```python
from build123d import *

# Parameters (mm, degrees)
SKETCH1_W           = 8.73
SKETCH1_H           = 8.73
BOSS_EXTRUDE1_DEPTH = 2.22
SKETCH2_R           = 25.695
BOSS_EXTRUDE2_DEPTH = 6
BOSS_EXTRUDE2_TAPER = 7
SKETCH3_R           = 23.86
CUT_EXTRUDE1_DEPTH  = 8.22
CUT_EXTRUDE1_DRAFT  = 7


with BuildPart() as part:
    # Sketch1 → Boss-Extrude1 (new body)
    with BuildSketch(Plane.XY):
        Polygon((-31.75, 0), (31.75, 0), (46.25, 25.11473671), (13.75, 81.406387956), (-13.75, 81.406387956), (-46.25, 25.11473671), align=None)
        Polygon((-34.392628869, 10.177167467), (-38.757628869, 17.737569242), (-31.197227094, 22.102569242), (-26.832227094, 14.542167467), align=None, mode=Mode.SUBTRACT)
        with Locations((0, 74.281387956)):
            Rectangle(SKETCH1_W, SKETCH1_H, mode=Mode.SUBTRACT)
        Polygon((34.392628869, 10.177167467), (38.757628869, 17.737569242), (31.197227094, 22.102569242), (26.832227094, 14.542167467), align=None, mode=Mode.SUBTRACT)
    extrude(amount=BOSS_EXTRUDE1_DEPTH)

    # Sketch2 → Boss-Extrude2 (add)
    with BuildSketch(Plane.XY.offset(2.22)):
        with Locations((0, 38)):
            Circle(SKETCH2_R)
    extrude(amount=BOSS_EXTRUDE2_DEPTH, taper=BOSS_EXTRUDE2_TAPER)


with BuildPart() as cut_extrude1_tool:
    # Sketch3 → Cut-Extrude1 (with draft: the straight prism first)
    with BuildSketch(Plane.XY.offset(8.22)):
        with Locations((0, 38)):
            Circle(SKETCH3_R)
    extrude(amount=-CUT_EXTRUDE1_DEPTH)
    # Cut-Extrude1: the draft: its side faces are tilted about the plane it starts from
    cut_extrude1_sides = [cut_extrude1_tool.faces().sort_by_distance(p)[0] for p in [
        (-23.86, 38, 4.11),
    ]]
    draft(cut_extrude1_sides, Plane.XY.offset(8.22), CUT_EXTRUDE1_DRAFT)


with BuildPart() as part_1:
    add(part.part)

    # Cut-Extrude1: cut by cut_extrude1_tool
    add(cut_extrude1_tool.part, mode=Mode.SUBTRACT)


solid = part_1.part
```
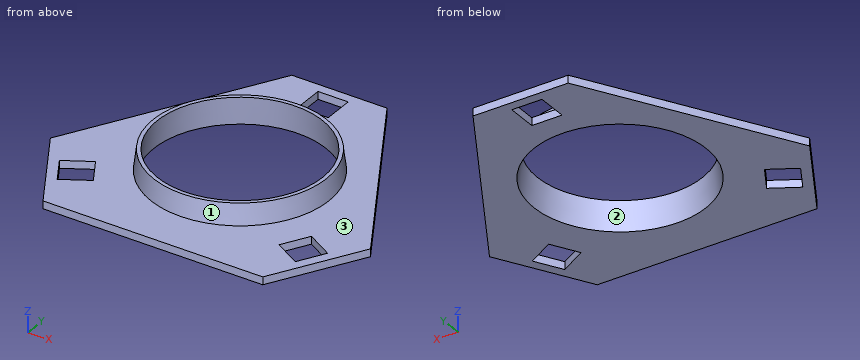
Could you check a few things on this model? Use its own coordinates, in mm. Face numbers are marked on the shaded views. Round coordinates to 2 decimals unless told otherwise and drop trailing zeros. Write each loop counter-clockwise with the first axis right and the second up, starting at its lowest first coordinate (ties: lowest second). Pieces come first, ordered by that corner, then holes.
(1) Suppose I cut it at D-D on z = 4.5. Write out the boundary of the cut face in (x, y).
Findings below:
outline: circle Ø50.83 at (0, 38); hole circle Ø48.63 at (0, 38)
(2) If I drill on probe 1 along X at (y, z) = (17.5, 1.75); probe 2 along Z at (x, y) = (17.5, 14); probe 3 along X at (y, z) = (22, 1.5), over which ranges is the centre line in solid material (lowest first)?
Findings below:
probe 1: x = -41.85 to -38.62, -28.54 to -13.7, 13.7 to 28.54, 38.62 to 41.85
probe 2: z = 0 to 2.22
probe 3: x = -44.45 to -31.37, -31.14 to -18.8, 18.8 to 31.14, 31.37 to 44.45
(3) Suppose I cut it at C-C on y = 38. Write out the boundary of the cut face in (x, z) (3 decimals), and give its area (3 significant figures).
Findings below:
outline: (-38.811, 0) - (-24.869, 0) - (-23.86, 8.22) - (-24.958, 8.22) - (-25.695, 2.22) - (-38.811, 2.22) - close; (23.86, 8.22) - (24.869, 0) - (38.811, 0) - (38.811, 2.22) - (25.695, 2.22) - (24.958, 8.22) - close
area: 75.7 mm2
(4) Suppose I cut it at A-A on x = 0. Write out the boundary of the cut face in (y, z) (3 decimals).
Findings below:
outline: (0, 0) - (13.131, 0) - (14.14, 8.22) - (13.042, 8.22) - (12.305, 2.22) - (0, 2.22) - close; (61.86, 8.22) - (62.869, 0) - (69.916, 0) - (69.916, 2.22) - (63.695, 2.22) - (62.958, 8.22) - close; (78.646, 0) - (81.406, 0) - (81.406, 2.22) - (78.646, 2.22) - close
(5) For pin 1 (1.1 mm diameter, centred on y = 75, z = 1, fed in from -X); pin 2 (8 mm diameter, centred on x = 30, y = 27, fed in from +Z); pin 3 (2.5 mm diameter, centred on y = 76, z = 1.5, fed in from +X), each with a flat end and sliding along its axis, tell me the tip position at first contact or that it passes through.
Findings below:
pin 1: stops at x = -17.77
pin 2: stops at z = 2.22
pin 3: stops at x = 17.59
(6) Thinking about a two-plate mould opening in X: for the marked faces 1, 2 and 3, which applies, +X half, -X half, draft (parallel to the pull), parting line (faces both ways), or undercut?
Findings below:
face 1: parting line
face 2: undercut
face 3: draft
(7) Suppose I cut it at B-B on x = 29.5. Write out the boundary of the cut face in (y, z), and give its area (3 significant figures).
Findings below:
outline: (0, 0) - (13, 0) - (13, 2.22) - (0, 2.22) - close; (19.16, 0) - (54.13, 0) - (54.13, 2.22) - (19.16, 2.22) - close
area: 106 mm2
